from build123d import *

# Parameters (mm, degrees)
SKETCH1_W                               = 152.4
SKETCH1_H                               = 152.4
BOSS_EXTRUDE1_DEPTH                     = 11.4
SKETCH5_W                               = 85
SKETCH5_H                               = 32
BOSS_EXTRUDE2_DEPTH                     = 10.2
SKETCH6_W                               = 32
SKETCH6_H                               = 85
BOSS_EXTRUDE3_DEPTH                     = 10.2
SKETCH7_W                               = 25.4
SKETCH7_H                               = 152.4
CUT_EXTRUDE1_DEPTH                      = 0.7
SKETCH8_W                               = 152.4
SKETCH8_H                               = 25.4
CUT_EXTRUDE2_DEPTH                      = 0.7
FILLET3_R                               = 15
M8X1_25_TAPPED_HOLE2_D                  = 6.8
F_10_32_TAPPED_HOLE3_D                  = 4.0386
F_10_32_TAPPED_HOLE3_DEPTH              = 9.38
F_10_32_TAPPED_HOLE3_TIP                = 1.213317848
F_10_32_TAPPED_HOLE4_D                  = 4.0386
F_10_32_TAPPED_HOLE4_DEPTH              = 9.38
F_10_32_TAPPED_HOLE4_TIP                = 1.213317848
M6X1_0_TAPPED_HOLE1_D                   = 5
M6X1_0_TAPPED_HOLE2_D                   = 5
CBORE_FOR_M8_HEX_HEAD_BOLT3_D           = 9
CBORE_FOR_M8_HEX_HEAD_BOLT3_CBORE_D     = 14
CBORE_FOR_M8_HEX_HEAD_BOLT3_CBORE_DEPTH = 10.18
CBORE_FOR_M8_HEX_HEAD_BOLT4_D           = 9
CBORE_FOR_M8_HEX_HEAD_BOLT4_CBORE_D     = 14
CBORE_FOR_M8_HEX_HEAD_BOLT4_CBORE_DEPTH = 10.18


with BuildPart() as part:
    # Sketch1 → Boss-Extrude1 (new body)
    with BuildSketch(Plane(origin=(0, 0, 0), x_dir=(1, 0, 0), z_dir=(0, 1, 0))):
        Rectangle(SKETCH1_W, SKETCH1_H)
    extrude(amount=BOSS_EXTRUDE1_DEPTH)

    # Sketch5 → Boss-Extrude2 (add)
    with BuildSketch(Plane(origin=(0, 11.4, 0), x_dir=(1, 0, 0), z_dir=(0, 1, 0))):
        with Locations((-33.7, 60.2)):
            Rectangle(SKETCH5_W, SKETCH5_H)
        with Locations((33.7, -60.2)):
            Rectangle(SKETCH5_W, SKETCH5_H)
    extrude(amount=BOSS_EXTRUDE2_DEPTH)

    # Sketch6 → Boss-Extrude3 (add)
    with BuildSketch(Plane.XZ):
        with Locations((60.2, 33.7)):
            Rectangle(SKETCH6_W, SKETCH6_H)
        with Locations((-60.2, -33.7)):
            Rectangle(SKETCH6_W, SKETCH6_H)
    extrude(amount=BOSS_EXTRUDE3_DEPTH)

    # Sketch7 → Cut-Extrude1 (cut)
    with BuildSketch(Plane.XZ):
        Rectangle(SKETCH7_W, SKETCH7_H)
    extrude(amount=-CUT_EXTRUDE1_DEPTH, mode=Mode.SUBTRACT)

    # Sketch8 → Cut-Extrude2 (cut)
    with BuildSketch(Plane(origin=(0, 11.4, 0), x_dir=(1, 0, 0), z_dir=(0, 1, 0))):
        Rectangle(SKETCH8_W, SKETCH8_H)
    extrude(amount=-CUT_EXTRUDE2_DEPTH, mode=Mode.SUBTRACT)

    # Fillet3
    fillet3_edges = [part.edges().sort_by_distance(p)[0] for p in [
        (76.2, 5.7, 76.2),
        (-76.2, 5.7, -76.2),
    ]]
    fillet(fillet3_edges, radius=FILLET3_R)

    # M8x1.25 Tapped Hole2 (through all)
    with Locations(Plane(origin=(0, -10.2, 0), x_dir=(-1, 0, 0), z_dir=(0, -1, 0))):
        with Locations((-61.7, -61.7), (61.7, 61.7)):
            Hole(M8X1_25_TAPPED_HOLE2_D / 2)

    # #10-32 Tapped Hole3
    with Locations(Plane(origin=(0, 11.4, 0), x_dir=(1, 0, 0), z_dir=(0, 1, 0))):
        with Locations((-21.2, -66.2), (-61.2, -66.2), (21.2, 66.2), (61.2, 66.2)):
            Hole(F_10_32_TAPPED_HOLE3_D / 2, depth=F_10_32_TAPPED_HOLE3_DEPTH)
            with Locations((0, 0, -(F_10_32_TAPPED_HOLE3_DEPTH + F_10_32_TAPPED_HOLE3_TIP / 2))):  # 118° drill point
                Cone(0, F_10_32_TAPPED_HOLE3_D / 2, F_10_32_TAPPED_HOLE3_TIP, mode=Mode.SUBTRACT)

    # #10-32 Tapped Hole4
    with Locations(Plane(origin=(0, 0, 0), x_dir=(-1, 0, 0), z_dir=(0, -1, 0))):
        with Locations((66.2, -61.2), (66.2, -21.2), (-66.2, 61.2), (-66.2, 21.2)):
            Hole(F_10_32_TAPPED_HOLE4_D / 2, depth=F_10_32_TAPPED_HOLE4_DEPTH)
            with Locations((0, 0, -(F_10_32_TAPPED_HOLE4_DEPTH + F_10_32_TAPPED_HOLE4_TIP / 2))):  # 118° drill point
                Cone(0, F_10_32_TAPPED_HOLE4_D / 2, F_10_32_TAPPED_HOLE4_TIP, mode=Mode.SUBTRACT)

    # M6x1.0 Tapped Hole1 (through all)
    with Locations(Plane(origin=(0, 10.7, 0), x_dir=(1, 0, 0), z_dir=(0, 1, 0))):
        with Locations((-60.2, 0)):
            Hole(M6X1_0_TAPPED_HOLE1_D / 2)

    # M6x1.0 Tapped Hole2 (through all)
    with Locations(Plane(origin=(0, 0.7, 0), x_dir=(-1, 0, 0), z_dir=(0, -1, 0))):
        with Locations((0, 60.2)):
            Hole(M6X1_0_TAPPED_HOLE2_D / 2)

    # CBORE for M8 Hex Head Bolt3 (through all)
    with Locations(Plane(origin=(0, -10.2, 0), x_dir=(-1, 0, 0), z_dir=(0, -1, 0))):
        with Locations((61.2, 20.2), (-61.2, -20.2)):
            CounterBoreHole(CBORE_FOR_M8_HEX_HEAD_BOLT3_D / 2, CBORE_FOR_M8_HEX_HEAD_BOLT3_CBORE_D / 2, CBORE_FOR_M8_HEX_HEAD_BOLT3_CBORE_DEPTH)

    # CBORE for M8 Hex Head Bolt4 (through all)
    with Locations(Plane(origin=(0, 21.6, 0), x_dir=(1, 0, 0), z_dir=(0, 1, 0))):
        with Locations((-20.2, 61.2), (20.2, -61.2)):
            CounterBoreHole(CBORE_FOR_M8_HEX_HEAD_BOLT4_D / 2, CBORE_FOR_M8_HEX_HEAD_BOLT4_CBORE_D / 2, CBORE_FOR_M8_HEX_HEAD_BOLT4_CBORE_DEPTH)


solid = part.part
Geometry: final body of the model. Coordinates: model frame, mm. A direction names the side the tool comes from. Round coordinates to 2 decimals unless told otherwise and drop trailing zeros. Loops run counter-clockwise (first coordinate to the right, second up) from the corner with the lowest first, then second, coordinate; pieces in that order, holes last.
Q1. Pin query (flat end, axial travel): P1, Ø2.5, axis at x = -66.2, z = 61.2, coming from the +Y side; P2, Ø7, axis at x = 20.2, z = 61.2, coming from the +Y side; P3, Ø8, axis at x = 40.5, y = 15.5, coming from the -Z side; P4, Ø1, axis at y = -5.5, z = 27, coming from the -X side. Return the tip coordinate at first contact, or that it passes through.
Q2. Section D-D on z = -37.5. Return loops of the section in (x, y).
Q3. Access query for faces 4 (the cylindrical face through (-22.132, 6.644, 67.991)), 5 (the flat face through (60, -5, -8.8)), 6 (the flat face through (8.8, 16, -60)), 7 (the flat face through (0, 0.7, 1)), 8 (the flat face through (-60, -5, 8.8)). Directions: +Z, -Z, +X, -X, +Y, -Y. A direction counts if a zero-diameter tool reaches every point of the face in a straight line with its end or side. Return the directions, or none.
Q4. Section B-B on x = 0. Return loops of the section in (y, z).
Q5. Section A-A on y = -3. Return loops of the section in (x, z), plus the area to 3 significant figures.
Q6. Material intervals for L1, parallel to Z at x = 21, y = 5; L2, parallel to Z at x = -20.2, y = 3.5; L3, parallel to Z at x = 61, y = 7, sorted ascending.
Q7. Pull-direction query (X, two-part tool) for faces 1 (the flat face through (-1, 10.7, 0)), 2 (the cylindrical face through (71.69, 5.92, 71.92)), 3 (the conical face through (-61.55, 1.017, 66.185)); classes: released by +X, released by -X, zero draft, split by the parting line, or undercut.
Q8. Section C-C on y = 7.5. State how many separate pieces and enclosed holes the cut face has, plus the area to 3 significant figures.
Evaluation:
1. P1: stops at y = 11.4
1. P2: passes through
1. P3: stops at z = 44.2
1. P4: stops at x = 44.2
2. outline: (-76.2, -10.2) - (-44.2, -10.2) - (-44.2, 0) - (-12.7, 0) - (-12.7, 0.7) - (12.7, 0.7) - (12.7, 0) - (76.2, 0) - (76.2, 11.4) - (-76.2, 11.4) - close
3. face 4: +Y
3. face 5: -Z, +X, -Y
3. face 6: -Z, +X, +Y
3. face 7: +Z, -Z, -Y
3. face 8: +Z, -X, -Y
4. outline: (0.7, -76.2) - (21.6, -76.2) - (21.6, -62.7) - (0.7, -62.7) - close; (0.7, -57.7) - (21.6, -57.7) - (21.6, -44.2) - (11.4, -44.2) - (11.4, -12.7) - (10.7, -12.7) - (10.7, 12.7) - (11.4, 12.7) - (11.4, 44.2) - (21.6, 44.2) - (21.6, 76.2) - (0.7, 76.2) - close
5. outline: (-76.2, -61.2) arc R15 ccw to (-61.2, -76.2) - (-44.2, -76.2) - (-44.2, 8.8) - (-76.2, 8.8) - close; (44.2, -8.8) - (76.2, -8.8) - (76.2, 61.2) arc R15 ccw to (61.2, 76.2) - (44.2, 76.2) - close; hole circle Ø14 at (-61.2, -20.2); hole circle Ø6.8 at (-61.7, -61.7); hole circle Ø5 at (-60.2, 0); hole circle Ø14 at (61.2, 20.2); hole circle Ø6.8 at (61.7, 61.7)
5. area: 4,940 mm2
6. L1: z = -76.2 to -68.21, -64.19 to 56.77, 65.63 to 76.2
6. L2: z = -76.2 to -65.7, -56.7 to 64.45, 67.95 to 76.2
6. L3: z = -76.2 to -68.21, -64.19 to 15.7, 24.7 to 58.37, 65.03 to 76.2
7. face 1: zero draft
7. face 2: released by +X
7. face 3: undercut
8. separate pieces: 1
8. enclosed holes: 16
8. area: 22,700 mm2
